Print and shaded views of the part. All mm, measured from the part's lowest x, y and z. Coordinates: 2 decimals unless noted, no trailing zeros. Loops run counter-clockwise (first coordinate to the right, second up) from the corner with the lowest first, then second, coordinate; pieces in that order, holes last.
1) Saw through at B-B, the plane z = 8. Write the cut outline in (x, y), and give its area (3 significant figures).
2) Two-plate mould, pull along Y, no slides. Class the marked faces 1, 2, 3 and 4: +Y half, -Y half, draft (parallel to the pull), parting line (faces both ways), or undercut.
3) Saw through at C-C, the plane z = 15. Write the cut outline in (x, y), and give its area (3 significant figures).
4) Saw through at D-D, the plane x = 8. Write the cut outline in (y, z), and give its area (3 significant figures).
5) Wall check: line 1 along Y through (x, z) = (30, 12.25); line 2 along X through (y, z) = (21, 7); line 3 along X through (y, z) = (44, 4.25). Give the ranges that are in metal, low to high.
6) Saw through at A-A, the plane y = 45. Write the cut outline in (x, z).
7) Pin check, flat tips, straight feed: pin 1 Ø6 at (x, y) = (9.5, 17) entering from -Z; pin 2 Ø8 at (x, y) = (30, 25) entering from -Z. Stop position of each tip, or through.
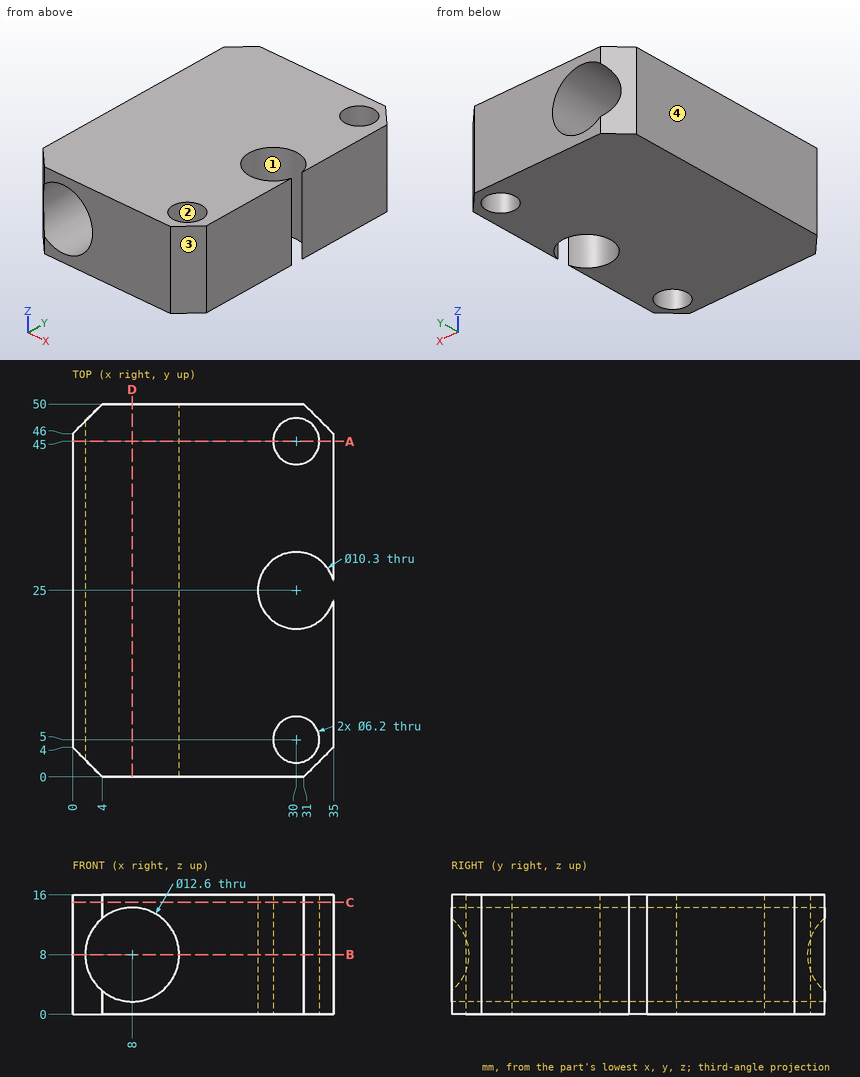
Data:
1. outline: (0, 4) - (1.7, 2.3) - (1.7, 47.7) - (0, 46) - close; (14.3, 0) - (31, 0) - (35, 4) - (35, 23.77) arc R5.15 cw (long way) to (35, 26.23) - (35, 46) - (31, 50) - (14.3, 50) - close; hole circle Ø6.2 at (30, 5); hole circle Ø6.2 at (30, 45)
1. area: 950 mm2
2. face 1: undercut
2. face 2: undercut
2. face 3: -Y half
2. face 4: draft
3. outline: (0, 4) - (4, 0) - (31, 0) - (35, 4) - (35, 23.77) arc R5.15 cw (long way) to (35, 26.23) - (35, 46) - (31, 50) - (4, 50) - (0, 46) - close; hole circle Ø6.2 at (30, 5); hole circle Ø6.2 at (30, 45)
3. area: 1,570 mm2
4. outline: (0, 0) - (50, 0) - (50, 1.7) - (0, 1.7) - close; (0, 14.3) - (50, 14.3) - (50, 16) - (0, 16) - close
4. area: 170 mm2
5. line 1: y = 0 to 1.9, 8.1 to 19.85, 30.15 to 41.9, 48.1 to 50
5. line 2: x = 0 to 1.78, 14.22 to 26.76, 33.24 to 35
5. line 3: x = 0 to 2.94, 13.06 to 27.07, 32.93 to 35
6. outline: (0, 0) - (26.9, 0) - (26.9, 16) - (0, 16) - close; (33.1, 0) - (35, 0) - (35, 16) - (33.1, 16) - close; hole circle Ø12.6 at (8, 8)
7. pin 1: stops at z = 0
7. pin 2: passes through
